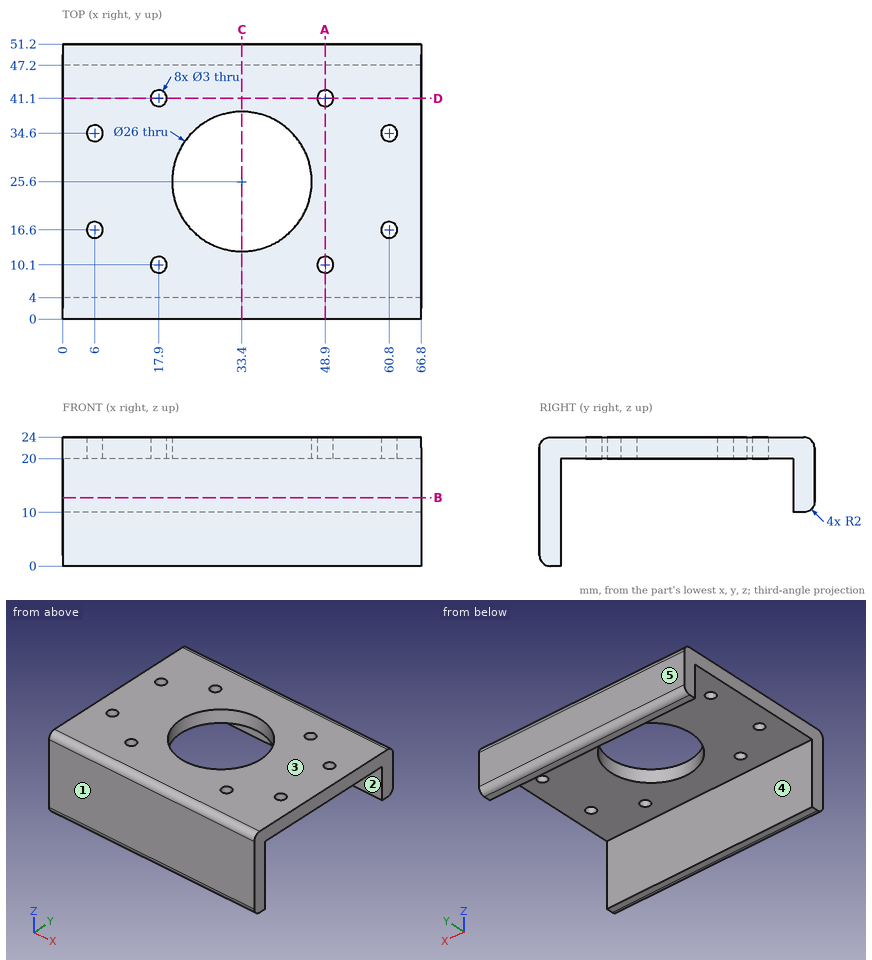
Check sheet for the drawn part. Datum: minimum x, y, z corner. Units: mm. A direction names the side the tool comes from. Round coordinates to 2 decimals unless told otherwise and drop trailing zeros. Order: outer loops, then holes, each group sorted by start corner. A loop starts at its lowest first (then second) coordinate and runs counter-clockwise, first axis right, second up. Notation, with made-up numbers: M 50.5,61 L 101.5,61 A3 ccw 101.5,65 Z; hole C 10,64.25 d11. An arc over 180 degrees is marked long. Answer in a Markdown table with one row per item.
(1) Set-up check for the marked faces 4 and 5: record each of +Z, -Z, +X, -X, +Y, -Y from which the full face is reachable in a straight line by a thin tool's end or side.
Findings:
| item | result |
|---|---|
| face 4 | -Z, +X, -X |
| face 5 | +Z, -Z, +X, -X, +Y |
(2) Section check C-C on x = 33.4. Record the boundary of the cut face in (y, z).
Findings:
| item | result |
|---|---|
| outline | M 0,2 A2 ccw 2,0 L 4,0 L 4,20 L 12.6,20 L 12.6,24 L 2,24 A2 ccw 0,22 Z; M 38.6,20 L 47.2,20 L 47.2,10 L 49.2,10 A2 ccw 51.2,12 L 51.2,22 A2 ccw 49.2,24 L 38.6,24 Z |
(3) Material ranges on line 1 along Y through (x, z) = (48.9, 21.65); line 2 along X through (y, z) = (41.1, 22.1); line 3 along Y through (x, z) = (14.5, 14.75), recorded low to high. Write a range as from..to.
Findings:
| item | result |
|---|---|
| line 1 | y = 0..8.6, 11.6..39.6, 42.6..51.2 |
| line 2 | x = 0..16.4, 19.4..47.4, 50.4..66.8 |
| line 3 | y = 0..4, 47.2..51.2 |
(4) Section check B-B on z = 12.75. Record the boundary of the cut face in (x, y).
Findings:
| item | result |
|---|---|
| outline | M 0,0 L 66.8,0 L 66.8,4 L 0,4 Z; M 0,47.2 L 66.8,47.2 L 66.8,51.2 L 0,51.2 Z |
(5) Gauge pin test, flat ends, axial feed: pin 1 (3.5 mm diameter, centred on x = 60.8, y = 16.6, fed in from -Z); pin 2 (1.6 mm diameter, centred on x = 49.5, y = 48, fed in from -Z); pin 3 (6 mm diameter, centred on x = 50, z = 5, fed in from +Y). Record the tip position at first contact, or that the pin passes through.
Findings:
| item | result |
|---|---|
| pin 1 | stops at z = 20 |
| pin 2 | stops at z = 10 |
| pin 3 | stops at y = 4 |
(6) Draft check along Y on the marked faces 1, 2 and 3. Enter one of: +Y half, -Y half, draft (parallel to the pull), parting line (faces both ways), or undercut.
Findings:
| item | result |
|---|---|
| face 1 | -Y half |
| face 2 | undercut |
| face 3 | draft |
(7) Section check D-D on y = 41.1. Record the boundary of the cut face in (x, z), plus the area to 3 significant figures.
Findings:
| item | result |
|---|---|
| outline | M 0,20 L 16.4,20 L 16.4,24 L 0,24 Z; M 19.4,20 L 47.4,20 L 47.4,24 L 19.4,24 Z; M 50.4,20 L 66.8,20 L 66.8,24 L 50.4,24 Z |
| area | 243 mm^2 |
(8) Section check A-A on x = 48.9. Record the boundary of the cut face in (y, z), plus the area to 3 significant figures.
Findings:
| item | result |
|---|---|
| outline | M 0,2 A2 ccw 2,0 L 4,0 L 4,20 L 8.6,20 L 8.6,24 L 2,24 A2 ccw 0,22 Z; M 11.6,20 L 39.6,20 L 39.6,24 L 11.6,24 Z; M 42.6,20 L 47.2,20 L 47.2,10 L 49.2,10 A2 ccw 51.2,12 L 51.2,22 A2 ccw 49.2,24 L 42.6,24 Z |
| area | 297 mm^2 |
